Design review of the part built by this model. Coordinates are the model's own, in mm. A direction names the side the tool comes from. Give positions to 0.01 mm unless a question says otherwise; leave off trailing zeros. Order: outer loops, then holes, each group sorted by start corner. A loop starts at its lowest first (then second) coordinate and runs counter-clockwise, first axis right, second up. Notation, with made-up numbers: (-5.5, 48.5) -> (36.5, 48.5) arc R10 cw to (36.5, 63.5) -> close; hole circle Ø5 at (-18.75, 69). An arc over 180 degrees is marked (long way). Use a Markdown table: item, result. Add a question column.
```python
from build123d import *

# Parameters (mm, degrees)
BOSS_EXTRUDE1_DEPTH      = 1100
BOSS_EXTRUDE1_DEPTH_BACK = 300
SKETCH1_R                = 7.5
CUT_EXTRUDE1_DEPTH       = 1142.753038095
CUT_EXTRUDE1_DEPTH_BACK  = 1142.753038095
SKETCH3_W                = 360
SKETCH3_H                = 60
SKETCH4_R                = 7.5
CUT_EXTRUDE2_DEPTH       = 1144.721994193
SKETCH7_W                = 25
SKETCH7_H                = 32
BOSS_EXTRUDE2_DEPTH      = 37.5
SKETCH8_W                = 16
SKETCH8_H                = 32.5
CUT_EXTRUDE4_DEPTH       = 1127.346305538
SKETCH9_W                = 16
SKETCH9_H                = 64
CUT_EXTRUDE5_DEPTH       = 24
SKETCH10_R               = 2.5908
CUT_EXTRUDE6_DEPTH       = 20


with BuildPart() as part:
    # Sketch1 → Boss-Extrude1 (new, two sides: drawn at the far end of the back side and taken through both)
    with BuildSketch(Plane.XY.offset(-BOSS_EXTRUDE1_DEPTH_BACK)):
        with BuildLine():
            Line((0, 0), (0, 30))
            Line((0, 30), (-300, 30))
            Line((-300, 30), (-300, 0))
            Line((-300, 0), (-300, -50))
            ThreePointArc((-300, -50), (-297.071067812, -57.071067812), (-290, -60))
            Line((-290, -60), (-285, -60))
            ThreePointArc((-285, -60), (-277.928932188, -57.071067812), (-275, -50))
            Line((-275, -50), (-275, 0))
            Line((-275, 0), (-25, 0))
            Line((-25, 0), (-25, -50))
            ThreePointArc((-25, -50), (-22.071067812, -57.071067812), (-15, -60))
            Line((-15, -60), (-10, -60))
            ThreePointArc((-10, -60), (-2.928932188, -57.071067812), (0, -50))
            Line((0, -50), (0, 0))
        make_face()
        with Locations((-12.5, -50)):
            Circle(SKETCH1_R, mode=Mode.SUBTRACT)
        with Locations(Location((-287.5, -50, 0), (0, 0, 180))):
            Circle(SKETCH1_R, mode=Mode.SUBTRACT)
    extrude(amount=BOSS_EXTRUDE1_DEPTH + BOSS_EXTRUDE1_DEPTH_BACK)

    # Sketch3 → Cut-Extrude1 (cut, two sides: drawn at the far end of the back side and taken through both)
    with BuildSketch(Plane(origin=(0, 0, 0), x_dir=(0, 0, -1), z_dir=(1, 0, 0)).offset(-CUT_EXTRUDE1_DEPTH_BACK)):
        with Locations((-920, -30)):
            Rectangle(SKETCH3_W, SKETCH3_H)
        Polygon((0, 0), (300, 0), (300, -60), (0, -60), (-60, -60), (-60, 0), align=None)
        Polygon((-690, -60), (-110, -60), (-110, -50), (-110, 0), (-690, 0), (-690, -50), align=None)
    extrude(amount=CUT_EXTRUDE1_DEPTH + CUT_EXTRUDE1_DEPTH_BACK, mode=Mode.SUBTRACT)

    # Sketch4 → Cut-Extrude2 (cut, through all)
    with BuildSketch(Plane(origin=(0, 30, 0), x_dir=(1, 0, 0), z_dir=(0, 1, 0))):
        with Locations(Location((-150, 0, 0), (0, 0, 180))):
            Circle(SKETCH4_R)
    extrude(amount=-CUT_EXTRUDE2_DEPTH, mode=Mode.SUBTRACT)

    # Sketch7 → Boss-Extrude2 (add)
    with BuildSketch(Plane(origin=(0, 0, 0), x_dir=(-1, 0, 0), z_dir=(0, -1, 0))):
        with Locations((150, 0)):
            Rectangle(SKETCH7_W, SKETCH7_H)
    extrude(amount=BOSS_EXTRUDE2_DEPTH)

    # Sketch8 → Cut-Extrude4 (cut, through all)
    with BuildSketch(Plane.XY.offset(16)):
        with Locations((-150, -16.25)):
            Rectangle(SKETCH8_W, SKETCH8_H)
    extrude(amount=-CUT_EXTRUDE4_DEPTH, mode=Mode.SUBTRACT)

    # Sketch9 → Cut-Extrude5 (cut)
    with BuildSketch(Plane.XZ):
        with Locations((-150, 0)):
            Rectangle(SKETCH9_W, SKETCH9_H)
    extrude(amount=-CUT_EXTRUDE5_DEPTH, mode=Mode.SUBTRACT)

    # Sketch10 → Cut-Extrude6 (cut)
    with BuildSketch(Plane(origin=(0, 30, 0), x_dir=(1, 0, 0), z_dir=(0, 1, 0))):
        with Locations(Location((-150, -1000, 0), (0, 0, 180))):
            Circle(SKETCH10_R)
        with Locations(Location((-162.7, -345.95, 0), (0, 0, 180))):
            Circle(SKETCH10_R)
        with Locations(Location((-137.3, -345.95, 0), (0, 0, 180))):
            Circle(SKETCH10_R)
    extrude(amount=-CUT_EXTRUDE6_DEPTH, mode=Mode.SUBTRACT)


solid = part.part
```
1) The part is to be moulded in two halves that separate along X. For faces 5 (the flat face through (-158, 2, 0)), 6 (the flat face through (-152, 15, 1100)), 7 (the flat face through (0, 7, 390)), say which applies: +X half, -X half, draft (parallel to the pull), parting line (faces both ways), or undercut.
2) For L1, parallel to Z at x = -150, y = 28.1; L2, parallel to X at y = 16, z = 345; L3, parallel to Y at x = -287, z = 87, list the stretches that pass through material, from the lowest coordinate up. Write a range as [from, to].
3) Machinability: for faces 1 (the flat face through (-13, -23, 690)), 2 (the flat face through (-288, -30, 60)), 3 (the flat face through (-13, -30, 740)), 4 (the flat face through (-275, -25, 715)), which of the approach directions +Z, -Z, +X, -X, +Y, -Y give a long, thin tool a straight path to every point of the face, cutting with its end or side? Answer none if there is none.
4) Insertion check: pin 1 (19.5 mm diameter, centred on x = -150, z = 0, fed in from +Y); pin 2 (8 mm diameter, centred on x = -148.5, z = 1, fed in from -Y); pin 3 (7.5 mm diameter, centred on x = -286, y = -22.5, fed in from -Z); pin 4 (8 mm diameter, centred on x = -176, y = -7, fed in from -Z). Each pin has a flat end and moves straight along its axis. Give the tip position at first contact, or say it passes through.
5) Add section A-A (z = -147.5). Give the boundary of the cut face in (x, y), then the cut area to 3 significant figures.
Worked answers:
| question | item | result |
|---|---|---|
| 1 | face 5 | undercut |
| 1 | face 6 | draft |
| 1 | face 7 | +X half |
| 2 | L1 | [-300, -7.5], [7.5, 997.41], [1002.59, 1100] |
| 2 | L2 | [-300, -165.11], [-160.29, -139.71], [-134.89, 0] |
| 2 | L3 | [-60, -57.48], [-42.52, 30] |
| 3 | face 1 | +X, -X, -Y |
| 3 | face 2 | -Z, +X, -X, -Y |
| 3 | face 3 | +Z, +X, -X, -Y |
| 3 | face 4 | +Z, -Z, -Y |
| 4 | pin 1 | y = 30 |
| 4 | pin 2 | y = -37.5 |
| 4 | pin 3 | z = 60 |
| 4 | pin 4 | through |
| 5 | outline | (-300, 0) -> (0, 0) -> (0, 30) -> (-300, 30) -> close |
| 5 | area | 9,000 mm^2 |
